Answer from the drawing. Dimensions are ordinates in mm from the lowest x, y and z of the part. A direction names the side the tool comes from. Coordinates: 2 decimals unless noted, no trailing zeros. Write each loop counter-clockwise with the first axis right and the second up, starting at its lowest first coordinate (ties: lowest second). Pieces come first, ordered by that corner, then holes. Notation, with made-up numbers: (32, 76) - (68, 76) arc R31 cw to (68, 103) - close; hole circle Ø7 at (14.5, 17). An arc over 180 degrees is marked (long way). Use a Markdown table: item, result.
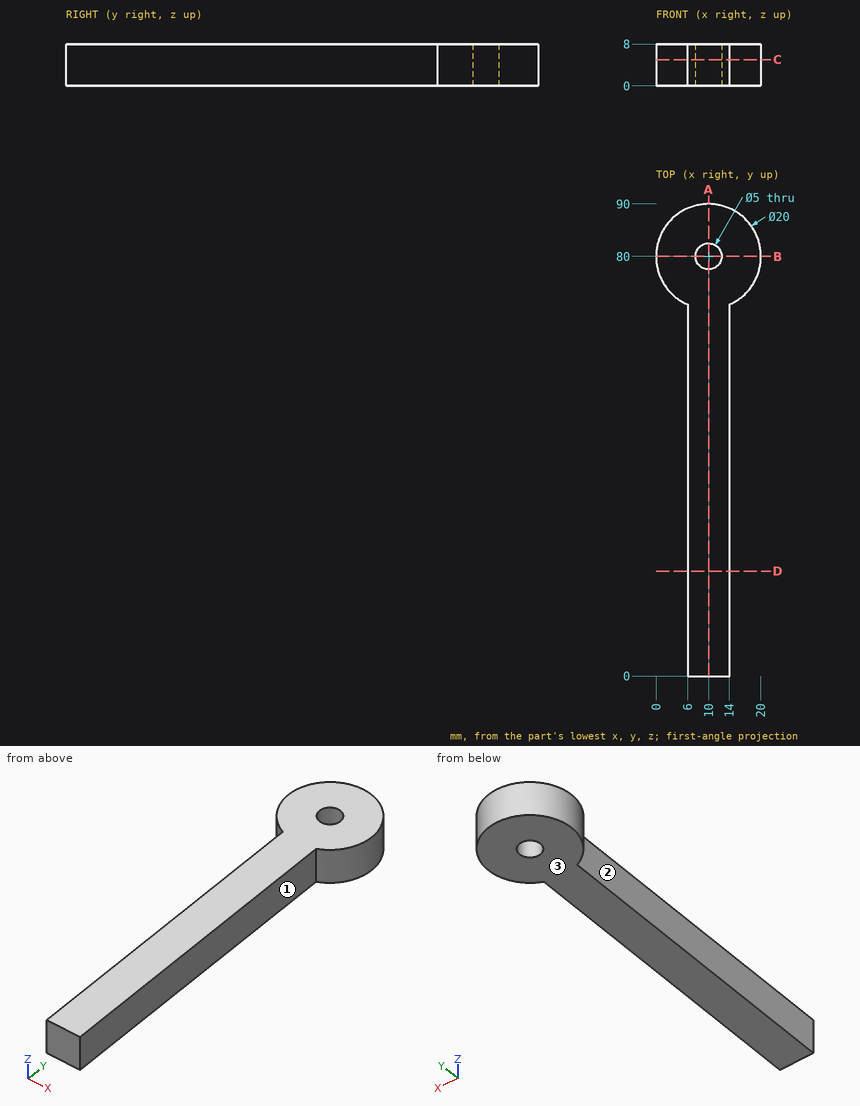
(1) Each of these flat-tipped pins is pushed along its axis until it touches: P1, Ø1, axis at x = 18, z = 6, coming from the +Y side; P2, Ø1.5, axis at y = 19, z = 5, coming from the +X side; P3, Ø2.5, axis at y = 43, z = 4.5, coming from the -X side. Where does it stop, or does it pass through?
Report:
| item | result |
|---|---|
| P1 | stops at y = 86.61 |
| P2 | stops at x = 14 |
| P3 | stops at x = 6 |
(2) A cutting plane is placed at C-C, the plane z = 5. Write down the section's boundary in (x, y).
Report:
| item | result |
|---|---|
| outline | (6, 0) - (14, 0) - (14, 70.83) arc R10 ccw (long way) to (6, 70.83) - close; hole circle Ø5 at (10, 80) |
(3) A cutting plane is placed at A-A, the plane x = 10. Write down the section's boundary in (y, z), and give its area (3 significant figures).
Report:
| item | result |
|---|---|
| outline | (0, 0) - (77.5, 0) - (77.5, 8) - (0, 8) - close; (82.5, 0) - (90, 0) - (90, 8) - (82.5, 8) - close |
| area | 680 mm² |
(4) A cutting plane is placed at B-B, the plane y = 80. Write down the section's boundary in (x, z).
Report:
| item | result |
|---|---|
| outline | (0, 0) - (7.5, 0) - (7.5, 8) - (0, 8) - close; (12.5, 0) - (20, 0) - (20, 8) - (12.5, 8) - close |
(5) For the marked faces 1, 2 and 3, determine the directions among +Z, -Z, +X, -X, +Y, -Y from which every point of the face is accessible in a straight line to the end or side of a thin tool.
Report:
| item | result |
|---|---|
| face 1 | +Z, -Z, +X, -Y |
| face 2 | +Z, -Z, -X, -Y |
| face 3 | -Z, +X, -X, +Y, -Y |
(6) A cutting plane is placed at D-D, the plane y = 20. Write down the section's boundary in (x, z), and give its area (3 significant figures).
Report:
| item | result |
|---|---|
| outline | (6, 0) - (14, 0) - (14, 8) - (6, 8) - close |
| area | 64.0 mm² |
(7) Straight lines are drawn through the part: L1, parallel to Y at x = 10, z = 5.5; L2, parallel to X at y = 51.5, z = 0.5; L3, parallel to Y at x = 12.25, z = 3. For each, find the intervals that lie inside material, in ascending order.
Report:
| item | result |
|---|---|
| L1 | y = 0 to 77.5, 82.5 to 90 |
| L2 | x = 6 to 14 |
| L3 | y = 0 to 78.91, 81.09 to 89.74 |
